Part model, mm, in its own coordinate system. A direction names the side the tool comes from. Coordinates: 2 decimals unless noted, no trailing zeros. Write each loop counter-clockwise with the first axis right and the second up, starting at its lowest first coordinate (ties: lowest second). Pieces come first, ordered by that corner, then holes. Notation, with made-up numbers: (40, 30.5) -> (69, 30.5) arc R25 cw to (69, 52.5) -> close; hole circle Ø8 at (74.5, 66). An arc over 180 degrees is marked (long way). One line per question, with ' | ' between items. Start each with the question number.
Item 1: Two-plate mould, pull along Z, no slides. Class faces 4 (the flat face through (22, -8, 0)), 5 (the flat face through (-27, -8, -5)), 6 (the flat face through (52, 6, -48)): pulls with the +Z half, pulls with the -Z half, needs draft (parallel to the pull), parting line crosses it, or undercut.
Item 2: Probe probe 1 along X at (y, z) = (1.7, 50); probe 2 along Z at (x, y) = (-50, 8.1). List the from-to ranges inside material, lowest first. Write a range as [from, to].
Item 3: Saw through at D-D (y = -1.5). List the corners of the cut face in (x, z).
Item 4: Pin check, flat tips, straight feed: pin 1 (2.5 mm diameter, centred on x = -27.5, y = -8.5, fed in from -Z); pin 2 (2.5 mm diameter, centred on y = -7.5, z = 1, fed in from -X); pin 3 (11 mm diameter, centred on x = -20, z = 37.5, fed in from -Y); pin 4 (3.5 mm diameter, centred on x = 50, z = 50, fed in from +Y) (3 decimals). Stop position of each tip, or through.
Item 5: Saw through at B-B (z = 0). List the corners of the cut face in (x, y).
Item 6: Saw through at A-A (x = 50). List the corners of the cut face in (y, z), and give its area (3 significant figures).
Item 7: Saw through at C-C (y = -9). List the corners of the cut face in (x, z).
Item 8: 3-axis set-ups, long thin cutter, end or side, ignore diameter. For faces 1 (the flat face through (-40, 2, -5)), 2 (the flat face through (-48, 6, -48)), 3 (the flat face through (32, -8, 0)): which of +Z, -Z, +X, -X, +Y, -Y reach the whole face in a straight line?
Autodesk Fusion 360 part; units mm, degrees
sketch "Sketch1" plane through (0, 0, 0) normal (0, 1, 0) x (1, 0, 0)
  line L0 (50, 50) -> (-50, 50)
  line L1 (-50, 50) -> (-50, -50)
  line L2 (-50, -50) -> (50, -50)
  line L3 (50, -50) -> (50, 50)
  line L4 (50, 50) -> (-50, -50) construction
  line L5 (-50, 50) -> (50, -50) construction
  circle A0 centre (-50, 50) radius 2.25
  circle A1 centre (50, 50) radius 2.25
  circle A2 centre (-50, -50) radius 2.25
  circle A3 centre (50, -50) radius 2.25
  line L6 (57.5, 57.5) -> (-57.5, 57.5)
  line L7 (-57.5, 57.5) -> (-57.5, -57.5)
  line L8 (-57.5, -57.5) -> (57.5, -57.5)
  line L9 (57.5, -57.5) -> (57.5, 57.5)
  line L10 (57.5, 57.5) -> (-57.5, -57.5) construction
  line L11 (-57.5, 57.5) -> (57.5, -57.5) construction
  circle A4 centre (-50, 50) radius 4
  circle A5 centre (50, 50) radius 4
  circle A6 centre (50, -50) radius 4
  circle A7 centre (-50, -50) radius 4
  dimension "d1" = 100
  dimension "d2" = 100
  dimension "d3" = 4.5
  dimension "d4" = 4.5
  dimension "d5" = 4.5
  dimension "d6" = 4.5
  dimension "d7" = 115
  dimension "d8" = 115
  dimension "d11" = 8
  dimension "d12" = 8
  dimension "d13" = 8
  dimension "d14" = 8
extrude "Extrude1" add sketch "Sketch1" along normal blind 10 contours L0 L1 A0 A4 | L0 L1 A0 A4 | L0 L1 L2 L3 A4 A5 A6 A7 | L0 L3 A1 A5 | L0 L3 A1 A5 | L1 L2 A2 A7 | L1 L2 A2 A7 | L2 L3 A3 A6 | L2 L3 A3 A6 | L6 L7 L8 L9
extrude "Extrude2" cut sketch "Sketch1" along normal blind 6 contours L0 L1 A0 A4 | L0 L1 A0 A4 | L0 L3 A1 A5 | L0 L3 A1 A5 | L1 L2 A2 A7 | L1 L2 A2 A7 | L2 L3 A3 A6 | L2 L3 A3 A6
sketch "Sketch2" plane through (0, 0, 0) normal (0, 1, 0) x (1, 0, 0)
  line L0 (57.5, 20) -> (-57.5, 20)
  line L1 (-57.5, 20) -> (-57.5, -20)
  line L2 (-57.5, -20) -> (57.5, -20)
  line L3 (57.5, -20) -> (57.5, 20)
  line L4 (57.5, 20) -> (-57.5, -20) construction
  line L5 (-57.5, 20) -> (57.5, -20) construction
  dimension "d17" = 115
  dimension "d18" = 40
extrude "Extrude3" add sketch "Sketch2" against normal blind 20
sketch "Sketch3" plane through (0, 10, 0) normal (0, 1, 0) x (-1, 0, 0)
  circle A0 centre (50, -50) radius 2.25
  circle A1 centre (-50, -50) radius 2.25
  circle A2 centre (-50, 50) radius 2.25
  circle A3 centre (50, 50) radius 2.25
  line L0 (-57.5, 57.5) -> (-57.5, -57.5)
  line L1 (-57.5, -57.5) -> (57.5, -57.5)
  line L2 (57.5, -57.5) -> (57.5, 57.5)
  line L3 (57.5, 57.5) -> (-57.5, 57.5)
  circle A4 centre (-40, 0) radius 7
  circle A5 centre (40, 0) radius 7
  circle A6 centre (40, 0) radius 4.25
  circle A7 centre (-40, 0) radius 4.25
  dimension "d21" = 14
  dimension "d22" = 14
  dimension "d23" = 8.5
  dimension "d24" = 8.5
extrude "Extrude4" cut sketch "Sketch3" against normal blind 8 contours A4 | A5
extrude "Extrude5" cut 2 faces at (-40.8833, 10, 1.9427) (39.1167, 10, 1.9427) along direction (0, -1, 0) blind 37
extrude "Extrude6" cut 1 faces at (-12.625, -20, 14.5602) along direction (0, 1, 0) blind 15
extrude "Extrude7" cut 1 faces at (-12.625, -5, 14.5602) along direction (0, 1, 0) blind 1
sketch "Sketch4" plane through (0, -4, 0) normal (0, -1, 0) x (1, 0, 0)
  circle A0 centre (-40, 0) radius 4.25
  circle A1 centre (40, 0) radius 4.25
  line L0 (57.5, -20) -> (57.5, 20)
  line L1 (57.5, 20) -> (-57.5, 20)
  line L2 (-57.5, 20) -> (-57.5, -20)
  line L3 (-57.5, -20) -> (57.5, -20)
  line L4 (-22, 5) -> (-32, 5)
  line L5 (-32, 5) -> (-32, -5)
  line L6 (-32, -5) -> (-22, -5)
  line L7 (-22, -5) -> (-22, 5)
  line L8 (-22, 5) -> (-32, -5) construction
  line L9 (-32, 5) -> (-22, -5) construction
  line L10 (0, 1.75) -> (0, 22.5)
  line L11 (22, 5) -> (32, 5)
  line L12 (32, 5) -> (32, -5)
  line L13 (32, -5) -> (22, -5)
  line L14 (22, -5) -> (22, 5)
  point P0 (-27, 0)
  dimension "d33" = 10
  dimension "d34" = 10
extrude "Extrude8" add sketch "Sketch4" along normal blind 8 contours L4 L5 L6 L7 | L11 L12 L13 L14
From the geometry:
1) face 4: needs draft | face 5: pulls with the -Z half | face 6: undercut
2) probe 1: [-57.5, -54], [-46, 46], [54, 57.5] | probe 2: [-57.5, -52.25], [-47.75, 47.75], [52.25, 57.5]
3) outline: (-57.5, -20) -> (57.5, -20) -> (57.5, 20) -> (-57.5, 20) -> close; hole circle Ø8.5 at (-40, 0); hole circle Ø8.5 at (40, 0)
4) pin 1: z = -5 | pin 2: x = -32 | pin 3: y = 0 | pin 4: through
5) outline: (-57.5, -4) -> (-44.25, -4) -> (-44.25, 2) -> (-47, 2) -> (-47, 10) -> (-57.5, 10) -> close; (-35.75, -4) -> (-32, -4) -> (-32, -12) -> (-22, -12) -> (-22, -4) -> (22, -4) -> (22, -12) -> (32, -12) -> (32, -4) -> (35.75, -4) -> (35.75, 2) -> (33, 2) -> (33, 10) -> (-33, 10) -> (-33, 2) -> (-35.75, 2) -> close; (44.25, -4) -> (57.5, -4) -> (57.5, 10) -> (47, 10) -> (47, 2) -> (44.25, 2) -> close
6) outline: (-4, -20) -> (0, -20) -> (0, -46) -> (6, -46) -> (6, -47.75) -> (10, -47.75) -> (10, 47.75) -> (6, 47.75) -> (6, 46) -> (0, 46) -> (0, 20) -> (-4, 20) -> close; (0, -57.5) -> (10, -57.5) -> (10, -52.25) -> (6, -52.25) -> (6, -54) -> (0, -54) -> close; (0, 54) -> (6, 54) -> (6, 52.25) -> (10, 52.25) -> (10, 57.5) -> (0, 57.5) -> close | area: 1,180 mm2
7) outline: (-32, -5) -> (-22, -5) -> (-22, 5) -> (-32, 5) -> close; (22, -5) -> (32, -5) -> (32, 5) -> (22, 5) -> close
8) face 1: +Y | face 2: -Y | face 3: +Z, -Z, +X, -Y
